Design review of the part built by this model. Coordinates are the model's own, in mm. A direction names the side the tool comes from. Coordinates: 2 decimals unless noted, no trailing zeros. Write each loop counter-clockwise with the first axis right and the second up, starting at its lowest first coordinate (ties: lowest second). Pieces come first, ordered by that corner, then holes. Notation, with made-up numbers: (24.25, 89.25) - (74.25, 89.25) arc R15 cw to (74.25, 108.25) - close; hole circle Ø11 at (-23, 73.25). An arc over 180 degrees is marked (long way). Answer as CSV lines item,"result". Start each with the question number.
Q1. We need section C-C (z = 1.45). State how many separate pieces and enclosed holes the cut face has, plus the area to 3 significant figures.
Q2. Clearance check with flat-ended pins moving along their axes: pin 1 (2.5 mm diameter, centred on y = 15.5, z = 2, fed in from -X); pin 2 (1.5 mm diameter, centred on y = 88.5, z = 2.5, fed in from -X); pin 3 (2.5 mm diameter, centred on y = 19, z = 2.5, fed in from -X). State where each tip first meets the part, or that it passes through.
Q3. We need section A-A (x = -138). Write out the cut boundary in (y, z).
Q4. We need section D-D (y = 37.5). Write out the cut boundary in (x, z).
Q5. Machinability: for faces 4 (the face through (-148, 102, 2)), 5 (the face through (-150.426, 87, 3)), which of the approach directions +Z, -Z, +X, -X, +Y, -Y give a long, thin tool a straight path to every point of the face, cutting with its end or side? Answer none if there is none.
Q6. Mouldability with a two-part tool opening along Y and no side actions: class faces 1 (the face through (-148, 61.1, 3)), 2 (the face through (-176.195, 2.258, 2.535)), 3 (the face through (-86, 0, 2)) as pulls with the +Y half, pulls with the -Y half, needs draft (parallel to the pull), parting line crosses it, or undercut.
Q7. We need section B-B (y = 48.5). Write out the cut boundary in (x, z).
Q8. For line 1 along Y through (x, z) = (-9, 3.8); line 2 along X through (y, z) = (32, 2); line 3 along X through (y, z) = (56, 4.05), list the stretches that pass through material, from the lowest coordinate up. Write a range as [from, to].
from build123d import *

# Parameters (mm, degrees)
SALIENTE_EXTRUIR1_DEPTH = 5
CORTAR_EXTRUIR3_DEPTH   = 10
REDONDEO4_R             = 2
CROQUIS3_W              = 5.2
CROQUIS3_H              = 8.2
CORTAR_EXTRUIR2_DEPTH   = 10
REDONDEO2_R             = 3
REDONDEO3_R             = 6
CROQUIS5_W              = 8.2
CROQUIS5_H              = 8.2
CORTAR_EXTRUIR4_DEPTH   = 10


with BuildPart() as part:
    # Croquis1 → Saliente-Extruir1 (new body)
    with BuildSketch(Plane.XY):
        with BuildLine():
            Line((0, 0), (-179.226162893, 0))
            Line((-179.226162893, 0), (-153.226162893, 102))
            Line((-153.226162893, 102), (-141.226162893, 102))
            Line((-141.226162893, 102), (-141.226162893, 77))
            ThreePointArc((-141.226162893, 77), (-81.241111145, 12.193748033), (-12, 67))
            Line((-12, 67), (0, 67))
            Line((0, 67), (0, 0))
        make_face()
    extrude(amount=SALIENTE_EXTRUIR1_DEPTH)

    # Croquis4 → Cortar-Extruir3 (cut)
    with BuildSketch(Plane.XY.offset(5)):
        Polygon((-166.357380645, 10), (-116.226162893, 10), (-157.435812017, 45), align=None)
        Polygon((-41.226162893, 10), (-26.226162893, 10), (-26.226162893, 22), align=None)
    extrude(amount=-CORTAR_EXTRUIR3_DEPTH, mode=Mode.SUBTRACT)

    # Redondeo4
    redondeo4_edges = [part.edges().sort_by_distance(p)[0] for p in [
        (-166.357380645, 10, 2.5),
        (-157.435812017, 45, 2.5),
        (-116.226162893, 10, 2.5),
        (-41.226162893, 10, 2.5),
        (-26.226162893, 22, 2.5),
        (-26.226162893, 10, 2.5),
    ]]
    fillet(redondeo4_edges, radius=REDONDEO4_R)

    # Croquis3 → Cortar-Extruir2 (cut)
    with BuildSketch(Plane.XY.offset(5)):
        with Locations((-147.826162893, 87)):
            Rectangle(CROQUIS3_W, CROQUIS3_H)
        with Locations((-147.826162893, 57)):
            Rectangle(CROQUIS3_W, CROQUIS3_H)
    extrude(amount=-CORTAR_EXTRUIR2_DEPTH, mode=Mode.SUBTRACT)

    # Redondeo2
    redondeo2_edges = [part.edges().sort_by_distance(p)[0] for p in [
        (0, 0, 2.5),
        (-153.226162893, 102, 2.5),
        (-141.226162893, 102, 2.5),
        (-12, 67, 2.5),
        (0, 67, 2.5),
    ]]
    fillet(redondeo2_edges, radius=REDONDEO2_R)

    # Redondeo3
    redondeo3_edges = [part.edges().sort_by_distance(p)[0] for p in [
        (-179.226162893, 0, 2.5),
    ]]
    fillet(redondeo3_edges, radius=REDONDEO3_R)

    # Croquis5 → Cortar-Extruir4 (cut)
    with BuildSketch(Plane.XY.offset(5)):
        with Locations((-7.1, 50)):
            Rectangle(CROQUIS5_W, CROQUIS5_H)
        with Locations((-7.1, 20)):
            Rectangle(CROQUIS5_W, CROQUIS5_H)
    extrude(amount=-CORTAR_EXTRUIR4_DEPTH, mode=Mode.SUBTRACT)


solid = part.part
Results list:
1,separate pieces,"1"
1,enclosed holes,"6"
1,area,"5,490 mm2"
2,pin 1,"stops at x = -175.59"
2,pin 2,"stops at x = -156.86"
2,pin 3,"stops at x = -174.7"
3,outline,"(0, 0) - (10, 0) - (10, 5) - (0, 5) - close; (28.49, 0) - (56.78, 0) - (56.78, 5) - (28.49, 5) - close"
4,outline,"(-169.67, 0) - (-159.35, 0) - (-159.35, 5) - (-169.67, 5) - close; (-148.61, 0) - (-127.85, 0) - (-127.85, 5) - (-148.61, 5) - close; (-24.6, 0) - (0, 0) - (0, 5) - (-24.6, 5) - close"
5,face 4,"+Z, -Z, +X, -X, +Y"
5,face 5,"+Z, -Z"
6,face 1,"undercut"
6,face 2,"parting line crosses it"
6,face 3,"pulls with the -Y half"
7,outline,"(-166.86, 0) - (-134.64, 0) - (-134.64, 5) - (-166.86, 5) - close; (-17.81, 0) - (-11.2, 0) - (-11.2, 5) - (-17.81, 5) - close; (-3, 0) - (0, 0) - (0, 5) - (-3, 5) - close"
8,line 1,"y = [0, 15.9], [24.1, 45.9], [54.1, 67]"
8,line 2,"x = [-171.07, -160.75], [-142.13, -123.13], [-29.32, 0]"
8,line 3,"x = [-164.95, -150.43], [-145.23, -137.74], [-14.71, 0]"
